Here's how the part is built. I have some questions about the finished solid (model axes, mm). A direction names the side the tool comes from. Round coordinates to 2 decimals unless told otherwise and drop trailing zeros. Loops run counter-clockwise (first coordinate to the right, second up) from the corner with the lowest first, then second, coordinate; pieces in that order, holes last. Notation, with made-up numbers: M -7,83 L 1,83 A11 ccw 1,91 Z; hole C 47,16 d5. An arc over 180 degrees is marked long. Write each question's results on one line, items separated by ' | '. Start each with the question number.
```python
from build123d import *

# Parameters (mm, degrees)
CHASIS_W                = 584.2
CHASIS_H                = 279.4
BOSS_EXTRUDE1_DEPTH     = 152.4
SKETCH3_W               = 44.45
SKETCH3_H               = 44.45
MIRROR2_COPY_1_SKETCH_W = 44.45
MIRROR2_COPY_1_SKETCH_H = 44.45


with BuildPart() as part:
    # Chasis → Boss-Extrude1 (new body)
    with BuildSketch(Plane(origin=(0, 0, 0), x_dir=(1, 0, 0), z_dir=(0, 1, 0))):
        Rectangle(CHASIS_W, CHASIS_H)
    extrude(amount=BOSS_EXTRUDE1_DEPTH)

    # Sketch3 → Revolve1 (revolve)
    with BuildSketch(Plane(origin=(0, 25.4, 0), x_dir=(-1, 0, 0), z_dir=(0, -1, 0))):
        with Locations((257.175, -98.425)):
            Rectangle(SKETCH3_W, SKETCH3_H)
    revolve1 = revolve(axis=Axis((-279.4, 25.4, 76.2), (1, 0, 0)))

    # Mirror1: Revolve1 across plane
    add(revolve1.mirror(Plane.XY))

    # Mirror2: Revolve1 across plane
    add(revolve1.mirror(Plane(origin=(0, 0, 0), x_dir=(0, 0, 1), z_dir=(1, 0, 0))))

    # Mirror2 copy 1 sketch → Mirror2 copy 1 (revolve)
    with BuildSketch(Plane.XZ.offset(-25.4)):
        with Locations((257.175, -98.425)):
            Rectangle(MIRROR2_COPY_1_SKETCH_W, MIRROR2_COPY_1_SKETCH_H)
    revolve(axis=Axis((279.4, 25.4, -76.2), (-1, 0, 0)))


solid = part.part
```
1. I want a section at A-A on z = 98. List the corners of the cut face in (x, y) for me.
2. If we mould it in two halves opening along Z, with no side actions, what happens to faces 1 (the face through (-4, 75, -139.7)), 2 (the face through (-257.486, -19.046, 76.799)), 3 (the face through (-279.4, -8, 76)), 4 (the face through (257.486, -19.046, 76.799))? For each: released by +Z, released by -Z, zero draft, split by the parting line, or undercut.
3. Which directions (+Z, -Z, +X, -X, +Y, -Y) give clear straight access to the entire face, cutting with the end or side of a thin tool? Please do faces 5 (the face through (234.95, -8, 76)), 6 (the face through (-4, 152.4, -2)), 7 (the face through (-292.1, 75, 2)), 8 (the face through (279.4, -8, 76)), 9 (the face through (-279.4, -8, -76)).
4. I want a section at B-B on x = 197. List the corners of the cut face in (y, z) for me, plus the area to 3 significant figures.
5. I need wall thicknesses on line 1 along Y through (x, z) = (7, 46.5); line 2 along X through (y, z) = (-4, 108.5); line 3 along Y through (x, z) = (251.5, -109.5). Which ranges of each line are inside material? Lowest first, please.
6. For pin 1 (15 mm diameter, centred on y = -12, z = 71.5, fed in from -X); pin 2 (15 mm diameter, centred on y = -11, z = -94, fed in from +X); pin 3 (3 mm diameter, centred on y = -2, z = 29, fed in from +X), each with a flat end and sliding along its axis, tell me the tip position at first contact or that it passes through.
7. I want a section at D-D on z = 5. List the corners of the cut face in (x, y) for me, plus the area to 3 significant figures.
8. I want a section at C-C on z = -97. List the corners of the cut face in (x, y) for me, plus the area to 3 significant figures.
Outcome:
1) outline: M -292.1,0 L -279.4,0 L -279.4,-13.34 L -234.95,-13.34 L -234.95,0 L 234.95,0 L 234.95,-13.34 L 279.4,-13.34 L 279.4,0 L 292.1,0 L 292.1,152.4 L -292.1,152.4 Z
2) face 1: released by -Z | face 2: undercut | face 3: zero draft | face 4: undercut
3) face 5: +Z, -Z, -Y | face 6: +Z, -Z, +X, -X, +Y | face 7: +Z, -Z, -X, +Y, -Y | face 8: +Z, -Z, +X, -Y | face 9: +Z, -Z, -X, -Y
4) outline: M 0,-139.7 L 152.4,-139.7 L 152.4,139.7 L 0,139.7 Z | area: 42,600 mm2
5) line 1: 0 to 152.4 | line 2: -279.4 to -234.95, 234.95 to 279.4 | line 3: -4.04 to 152.4
6) pin 1: x = -279.4 | pin 2: x = 279.4 | pin 3: through
7) outline: M -292.1,0 L 292.1,0 L 292.1,152.4 L -292.1,152.4 Z | area: 89,000 mm2
8) outline: M -292.1,0 L -279.4,0 L -279.4,-13.88 L -234.95,-13.88 L -234.95,0 L 234.95,0 L 234.95,-13.88 L 279.4,-13.88 L 279.4,0 L 292.1,0 L 292.1,152.4 L -292.1,152.4 Z | area: 90,300 mm2
